The listing builds one solid part. Answer for the finished solid, in the listing's coordinates (mm). Round coordinates to 2 decimals unless told otherwise and drop trailing zeros. Order: outer loops, then holes, each group sorted by start corner. A loop starts at its lowest first (then second) coordinate and runs counter-clockwise, first axis right, second up. Notation, with made-up numbers: (-31, 63.5) - (27, 63.5) arc R28 ccw to (27, 83.5) - close; hole circle Ø4 at (-27.75, 11.5). An arc over 180 degrees is marked (long way). Write item = value, one per line.
from build123d import *

# Parameters (mm, degrees)
SKETCH1_W           = 140
SKETCH1_H           = 40
SKETCH1_R           = 3
BOSS_EXTRUDE1_DEPTH = 3
FILLET1_R           = 0.5


with BuildPart() as part:
    # Sketch1 → Boss-Extrude1 (new, symmetric)
    with BuildSketch(Plane(origin=(0, 0, 0), x_dir=(1, 0, 0), z_dir=(0, 1, 0))):
        Rectangle(SKETCH1_W, SKETCH1_H)
        with Locations(Location((-40, 0, 0), (0, 0, 270))):
            Circle(SKETCH1_R, mode=Mode.SUBTRACT)
        with Locations(Location((-60, 0, 0), (0, 0, 270))):
            Circle(SKETCH1_R, mode=Mode.SUBTRACT)
    extrude(amount=BOSS_EXTRUDE1_DEPTH, both=True)

    # Fillet1
    fillet1_edges = [part.edges().sort_by_distance(p)[0] for p in [
        (-40, 3, -3),
        (-60, 3, -3),
    ]]
    fillet(fillet1_edges, radius=FILLET1_R)


solid = part.part
Q1. Determine the mould class of faces 1 (the face through (-37.47, -0.29, 1.61)), 2 (the face through (-1, -3, 0)), 3 (the face through (-1, 0, -20)) for opening direction Z: released by +Z, released by -Z, zero draft, split by the parting line, or undercut.
Model answer:
face_1 = undercut
face_2 = zero draft
face_3 = released by -Z
Q2. Section A-A on z = 0 is taken. Determine the outline of the cut face in (x, y).
Model answer:
outline = (-70, -3) - (-63, -3) - (-63, 2.5) arc R0.5 ccw to (-63.5, 3) - (-70, 3) - close; (-57, -3) - (-43, -3) - (-43, 2.5) arc R0.5 ccw to (-43.5, 3) - (-56.5, 3) arc R0.5 ccw to (-57, 2.5) - close; (-37, -3) - (70, -3) - (70, 3) - (-36.5, 3) arc R0.5 ccw to (-37, 2.5) - close
Q3. A flat-ended cylindrical pin translates along its axis: P1, Ø3.5, axis at x = -40, z = 0, coming from the -Y side. Find the tip coordinate at first contact, or state that the pin passes through.
Model answer:
P1 = through
Q4. Section B-B on x = -60 is taken. Determine the outline of the cut face in (y, z), then the cut area to 3 significant figures.
Model answer:
outline = (-3, -20) - (3, -20) - (3, -3.5) arc R0.5 ccw to (2.5, -3) - (-3, -3) - close; (-3, 3) - (2.5, 3) arc R0.5 ccw to (3, 3.5) - (3, 20) - (-3, 20) - close
area = 204 mm^2
Q5. Find the intervals of material crossed by line 1 (X direction, y = -0.65, z = 0); line 2 (X direction, y = -1.6, z = -1.5), in increasing order. Write a range as from..to.
Model answer:
line_1 = -70..-63, -57..-43, -37..70
line_2 = -70..-62.6, -57.4..-42.6, -37.4..70
